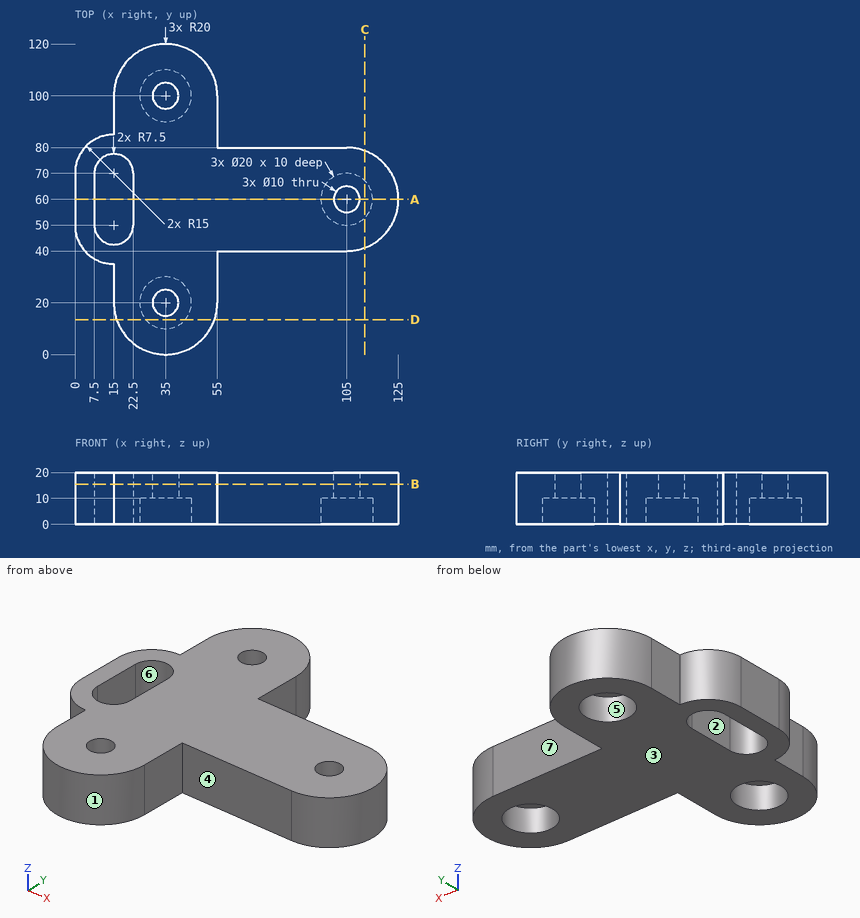
The drawing under review shows one solid part. Ordinate dimensions are in mm from its lowest x, y, z. A direction names the side the tool comes from. Round coordinates to 2 decimals unless told otherwise and drop trailing zeros. Write each loop counter-clockwise with the first axis right and the second up, starting at its lowest first coordinate (ties: lowest second). Pieces come first, ordered by that corner, then holes. Notation, with made-up numbers: (36.5, 2) -> (53.5, 2) arc R29 ccw to (53.5, 31) -> close; hole circle Ø10 at (89, 24.25). An arc over 180 degrees is marked (long way). One line per question, with ' | ' between items. Start each with the question number.
(1) Tool access review of the marked faces 4, 5, 6 and 7: name each direction out of +Z, -Z, +X, -X, +Y, -Y from which nothing blocks a thin tool from reaching the whole face with its end or side.
(2) Add section C-C, the plane x = 112. Write out the cut boundary in (y, z) (3 decimals).
(3) For line 1 along Y through (x, z) = (35, 16); line 2 along Y through (x, z) = (35, 6.25); line 3 along Y through (x, z) = (105, 6.5), list the stretches that pass through material, from the lowest coordinate up. Write a range as from..to.
(4) Mouldability with a two-part tool opening along Y and no side actions: class the marked faces 1, 2 and 3 as released by +Y, released by -Y, zero draft, split by the parting line, or undercut.
(5) Insertion check: P1, Ø6, axis at y = 79, z = 4, coming from the +X side; P2, Ø10, axis at y = 34.5, z = 7.5, coming from the +X side; P3, Ø1.5, axis at x = 42, z = 8.5, coming from the +Y side. Each pin has a flat end and moves straight along its axis. Give the tip position at first contact, or say it passes through.
(6) Add section D-D, the plane y = 13.5. Write out the cut boundary in (x, z), plus the area to 3 significant figures.
(7) Add section A-A, the plane y = 60. Write out the cut boundary in (x, z), plus the area to 3 significant figures.
(8) Add section B-B, the plane z = 15.5. Write out the cut boundary in (x, y), plus the area to 3 significant figures.
Answer list:
1) face 4: +Z, -Z, +X, -Y | face 5: -Z | face 6: +Z, -Z | face 7: +Z, -Z, +X, +Y
2) outline: (41.265, 0) -> (52.859, 0) -> (52.859, 10) -> (67.141, 10) -> (67.141, 0) -> (78.735, 0) -> (78.735, 20) -> (41.265, 20) -> close
3) line 1: 0..15, 25..95, 105..120 | line 2: 0..10, 30..90, 110..120 | line 3: 40..50, 70..80
4) face 1: released by -Y | face 2: undercut | face 3: zero draft
5) P1: x = 117 | P2: x = 55 | P3: y = 119
6) outline: (16.09, 0) -> (27.4, 0) -> (27.4, 10) -> (42.6, 10) -> (42.6, 0) -> (53.91, 0) -> (53.91, 20) -> (16.09, 20) -> close | area: 605 mm²
7) outline: (0, 0) -> (7.5, 0) -> (7.5, 20) -> (0, 20) -> close; (22.5, 0) -> (95, 0) -> (95, 10) -> (100, 10) -> (100, 20) -> (22.5, 20) -> close; (110, 10) -> (115, 10) -> (115, 0) -> (125, 0) -> (125, 20) -> (110, 20) -> close | area: 1,900 mm²
8) outline: (0, 50) arc R15 ccw to (15, 35) -> (15, 20) arc R20 ccw to (55, 20) -> (55, 40) -> (105, 40) arc R20 ccw to (105, 80) -> (55, 80) -> (55, 100) arc R20 ccw to (15, 100) -> (15, 85) arc R15 ccw to (0, 70) -> close; hole (7.5, 50) arc R7.5 ccw to (22.5, 50) -> (22.5, 70) arc R7.5 ccw to (7.5, 70) -> close; hole circle Ø10 at (35, 20); hole circle Ø10 at (35, 100); hole circle Ø10 at (105, 60) | area: 7,030 mm²
